Autodesk Inventor part; units mm, degrees
ref_plane "YZ Plane" through (0, 0, 0) normal (1, 0, 0) x (0, 1, 0)
ref_plane "XZ Plane" through (0, 0, 0) normal (0, 1, 0) x (-1, 0, 0)
ref_plane "XY Plane" through (0, 0, 0) normal (0, 0, 1) x (1, 0, 0)
sketch "Sketch1" plane through (0, 0, 0) normal (0, 1, 0) x (-1, 0, 0)
  circle A0 centre (0, 0) radius 5
  dimension "Diameter" = 10
extrude "Extrusion1" add sketch "Sketch1" along normal mid plane 6
sketch "Sketch2" plane through (0, 3, 0) normal (0, 1, 0) x (1, 0, 0)
  circle A0 centre (0, 0) radius 1.5
  dimension "d3" = 3
extrude "Extrusion2" cut sketch "Sketch2" against normal through all
sketch "Sketch3" plane through (0, 0, 0) normal (1, 0, 0) x (0, 1, 0)
  circle A0 centre (0, 0) radius 1.25
  dimension "d6" = 2.5
extrude "Extrusion3" cut sketch "Sketch3" against normal blind 6
chamfer "Chamfer1" distance 0.5 angle 45 2 edges at (5, 3, 0) (5, -3, 0)
chamfer "Chamfer2" distance 0.2 angle 45 2 edges at (-1.5, 3, 0) (-1.5, -3, 0)
thread "Thread1"
sketch "Sketch4" plane through (0, 3, 0) normal (0, 1, 0) x (1, 0, 0)
  point P0 (0, 0)
  point P1 (0, -3)
  dimension "d17" = 3
hole "Hole1" at (0, 3, 3) direction (0, -1, 0) diameter 0.5 end through all
properties part number "Pendulum Arm Cap" material "Stainless Steel"
Source: CAD feature listing. Evaluate the final solid. Frame: model axes, mm. Round coordinates to 2 decimals unless told otherwise and drop trailing zeros. Order: outer loops, then holes, each group sorted by start corner. A loop starts at its lowest first (then second) coordinate and runs counter-clockwise, first axis right, second up. Notation, with made-up numbers: (-14, -18) -> (-1, -18) arc R23 ccw to (-1, 5) -> close; hole circle Ø4 at (15.25, -18.75). An arc over 180 degrees is marked (long way). One line per item, written item: value. Start each with the question number.
Q1. Section query D-D (y = -1.65). Return the cut outline in (x, z).
Q2. Material intervals for probe 1 along Z at (x, y) = (0, -0.4); probe 2 along Z at (x, y) = (-4, 0), sorted ascending.
Q3. Pin query (flat end, axial travel): pin 1 (1.5 mm diameter, centred on x = 1.5, y = -2.5, fed in from -Z); pin 2 (2 mm diameter, centred on y = 0, z = 0, fed in from -X); pin 3 (1.5 mm diameter, centred on x = -2.5, y = -1, fed in from -Z). Return the tip coordinate at first contact, or that it passes through.
Q4. Section query B-B (x = 0). Return the cut outline in (y, z).
Q5. Section query C-C (y = 0). Return the cut outline in (x, z), plus the area to 3 significant figures.
Q6. Draft query along Z for faces 1 (the cylindrical face through (-2.885, 1.155, -0.479)), 2 (the cylindrical face through (1.08, -0.04, 4.88)), 3 (the flat face through (0, 3, -2)). Return one class per face: pulls with the +Z half, pulls with the -Z half, needs draft (parallel to the pull), parting line crosses it, or undercut.
Q7. Section query A-A (z = 0). Return the cut outline in (x, y).
Findings below:
1. outline: circle Ø10 at (0, 0); hole circle Ø3 at (0, 0); hole circle Ø0.5 at (0, 3)
2. probe 1: -5 to -1.5, 1.5 to 2.75, 3.25 to 5
2. probe 2: -3 to -1.25, 1.25 to 3
3. pin 1: z = -4.94
3. pin 2: x = 1.12
3. pin 3: z = -4.68
4. outline: (-3, -4.5) -> (-2.5, -5) -> (2.5, -5) -> (3, -4.5) -> (3, -1.7) -> (2.8, -1.5) -> (-2.8, -1.5) -> (-3, -1.7) -> close; (-3, 1.7) -> (-2.8, 1.5) -> (2.8, 1.5) -> (3, 1.7) -> (3, 2.75) -> (-3, 2.75) -> close; (-3, 3.25) -> (3, 3.25) -> (3, 4.5) -> (2.5, 5) -> (-2.5, 5) -> (-3, 4.5) -> close
5. outline: (-4.84, -1.25) arc R5 ccw (long way) to (-4.84, 1.25) -> (-0.83, 1.25) arc R1.5 cw (long way) to (-0.83, -1.25) -> close; hole circle Ø0.5 at (0, 3)
5. area: 62.2 mm²
6. face 1: undercut
6. face 2: parting line crosses it
6. face 3: needs draft
7. outline: (-5, -2.5) -> (-4.5, -3) -> (-1.7, -3) -> (-1.5, -2.8) -> (-1.5, -1.25) -> (-5, -1.25) -> close; (-5, 1.25) -> (-1.5, 1.25) -> (-1.5, 2.8) -> (-1.7, 3) -> (-4.5, 3) -> (-5, 2.5) -> close; (1.5, -2.8) -> (1.7, -3) -> (4.5, -3) -> (5, -2.5) -> (5, 2.5) -> (4.5, 3) -> (1.7, 3) -> (1.5, 2.8) -> close
